Autodesk Inventor part; units mm, degrees
ref_plane "YZ Plane" through (0, 0, 0) normal (1, 0, 0) x (0, 1, 0)
ref_plane "XZ Plane" through (0, 0, 0) normal (0, 1, 0) x (-1, 0, 0)
ref_plane "XY Plane" through (0, 0, 0) normal (0, 0, 1) x (1, 0, 0)
sketch "Sketch1" plane through (0, 0, 0) normal (0, 1, 0) x (-1, 0, 0)
  line L0 (275, 0) -> (-275, 0)
  arc A0 (-275, 0) -> (-275, -360) centre (82.2114, -180) ccw
  arc A1 (-275, -720) -> (-275, -360) centre (-632.2114, -540) ccw
  arc A2 (-275, -720) -> (-275, -1080) centre (82.2114, -900) ccw
  arc A3 (-275, -1440) -> (-275, -1080) centre (-632.2114, -1260) ccw
  line L1 (-275, -1440) -> (275, -1440)
  line L2 (0, 0) -> (0, -1440) construction
  arc A4 (275, 0) -> (275, -360) centre (632.2114, -180) ccw
  arc A5 (275, -720) -> (275, -360) centre (-82.2114, -540) ccw
  arc A6 (275, -720) -> (275, -1080) centre (632.2114, -900) ccw
  arc A7 (275, -1440) -> (275, -1080) centre (-82.2114, -1260) ccw
  arc A8 (255, 0) -> (255, -360) centre (612.2114, -180) ccw
  arc A9 (255, -720) -> (255, -360) centre (-102.2114, -540) ccw
  arc A10 (255, -720) -> (255, -1080) centre (612.2114, -900) ccw
  arc A11 (255, -1440) -> (255, -1080) centre (-102.2114, -1260) ccw
  arc A12 (-255, 0) -> (-255, -360) centre (102.2114, -180) ccw
  arc A13 (-255, -720) -> (-255, -360) centre (-612.2114, -540) ccw
  arc A14 (-255, -720) -> (-255, -1080) centre (102.2114, -900) ccw
  arc A15 (-255, -1440) -> (-255, -1080) centre (-612.2114, -1260) ccw
  point P0 (255, 0)
  point P1 (-255, 0)
  dimension "d10" = 550
  dimension "d11" = 360
  dimension "d12" = 550
  dimension "d13" = 360
  dimension "d14" = 360
  dimension "d15" = 360
  dimension "d16" = 400
  dimension "d26" = 20
  dimension "d27" = 20
extrude "Extrusion1" add sketch "Sketch1" along normal blind 3
extrude "Extrusion2" add sketch "Sketch1" along normal blind 3.1 contours A4 A5 A6 A7 L1 A11 A10 A9 A8 L0 | A12 A13 A14 A15 L1 A3 A2 A1 A0 L0
equation "\"d10\" = track_width"
equation "\"d12\" = d10"
equation "\"d13\" = d11"
equation "\"d14\" = d11"
equation "\"d15\" = d11"
equation "\"d26\" = d27"
equation "\"d27\" = curb_width"
equation "\"d22\" = track_height"
equation "\"d28\" = track_height + curb_height"
properties part number "chicane"
Input: part model. Units: mm. Frame: model coordinates. Give positions to 0.01 mm unless a question says otherwise; leave off trailing zeros. Loops run counter-clockwise (first coordinate to the right, second up) from the corner with the lowest first, then second, coordinate; pieces in that order, holes last. Notation, with made-up numbers: M 67,-19 L 110,-19 A5 cw 110,-12 Z; hole C -32,-20.5 d4. An arc over 180 degrees is marked long. Use one line per item in the form item = value.
1. Section query B-B, the plane z = -1043. Return the cut outline in (x, y).
Numbers:
outline = M -258.65,0 L 291.35,0 L 291.35,3.1 L 271.35,3.1 L 271.35,3 L -238.65,3 L -238.65,3.1 L -258.65,3.1 Z
2. Line query: L1, parallel to Y at x = 115.5, z = -803; L2, parallel to X at y = 2.8, z = -851.5; L3, parallel to X at y = 2.5, z = -940. Output: solid intervals per line, ascending.
Numbers:
L1 = 0 to 3
L2 = -235.16 to 314.84
L3 = -234.22 to 315.78
3. Section query C-C, the plane x = 69. Return the cut outline in (y, z).
Numbers:
outline = M 0,-1440 L 3,-1440 L 3,0 L 0,0 Z
4. Section query A-A, the plane y = 2.25. Return the cut outline in (x, z).
Numbers:
outline = M -275,-1440 L 275,-1440 A400 cw 275,-1080 A400 ccw 275,-720 A400 cw 275,-360 A400 ccw 275,0 L -275,0 A400 cw -275,-360 A400 ccw -275,-720 A400 cw -275,-1080 A400 ccw Z
5. First-contact query: pin 1 (6 mm diameter, centred on x = 160, z = -1223, fed in from +Y). Flat tip, straight axial feed; report the tip coordinate or a pass-through.
Numbers:
pin_1 = 3
